Autodesk Inventor part; units mm, degrees
ref_plane "YZ Plane" through (0, 0, 0) normal (1, 0, 0) x (0, 1, 0)
ref_plane "XZ Plane" through (0, 0, 0) normal (0, 1, 0) x (-1, 0, 0)
ref_plane "XY Plane" through (0, 0, 0) normal (0, 0, 1) x (1, 0, 0)
sketch "Skizze1" plane through (0, 0, 0) normal (0, 0, 1) x (1, 0, 0)
  line L0 (11.5, 38) -> (-11.5, 38)
  line L1 (-11.5, 38) -> (-11.5, -38)
  line L2 (-11.5, -38) -> (11.5, -38)
  line L3 (11.5, -38) -> (11.5, 38)
  line L4 (11.5, 38) -> (-11.5, -38) construction
  line L5 (-11.5, 38) -> (11.5, -38) construction
  line L6 (-23, -50) -> (23, -50)
  line L7 (23, -50) -> (23, -38)
  line L8 (23, -38) -> (-23, -38)
  line L9 (-23, -38) -> (-23, -50)
  line L10 (-23, -50) -> (23, -38) construction
  line L11 (23, -50) -> (-23, -38) construction
  line L12 (-23, -38) -> (-11.5, -38)
  line L13 (-11.5, -38) -> (-11.5, 12)
  line L14 (-11.5, 12) -> (-23, 12)
  line L15 (-23, 12) -> (-23, -38)
  line L16 (23, -38) -> (11.5, -38)
  line L17 (11.5, -38) -> (11.5, 12)
  line L18 (11.5, 12) -> (23, 12)
  line L19 (23, 12) -> (23, -38)
  point P0 (0, 0)
  point P1 (0, -44)
  point P2 (0, -38)
  dimension "d0" = 23
  dimension "d1" = 76
  dimension "d2" = 12
  dimension "d3" = 50
  dimension "d4" = 50
  dimension "d5" = 46
extrude "Extrusion1" add sketch "Skizze1" along normal blind 10 contours L18 L19 L8 L3 | L1 L8 L15 L14 | L8 L7 L6 L9 L2
sketch "Skizze2" plane through (-11.5, -38, 0) normal (1, 0, 0) x (0, 0, -1)
  line L0 (0, 50) -> (0, -12)
  line L1 (0, -7.7211) -> (-0.5, -7.7211)
  line L2 (-0.5, -7.7211) -> (-2, -3.621)
  line L3 (-2, -3.621) -> (-2, 50)
  line L4 (-2, 50) -> (0, 50)
  line L5 (0, 0) -> (0, 50)
  point P0 (0, 38)
  point P1 (0, 5.0638)
  dimension "d8" = 0.5
  dimension "d15" = 2
extrude "Extrusion2" cut sketch "Skizze2" along normal blind 25 and the other way blind 2
sketch "Skizze3" plane through (-23, -50, 0) normal (-1, 0, 0) x (0, 0, 1)
  line L0 (0, 62) -> (0, 0)
  line L1 (0, 0) -> (10, 0)
  line L2 (10, 62) -> (10, 0)
  line L3 (0, 62) -> (10, 62)
  circle A0 centre (6.7241, 56.1881) radius 1.5
  point P0 (0, 50)
  dimension "d11" = 3
extrude "Extrusion3" cut sketch "Skizze3" against normal through all contours A0
fillet "Rundung1" radius 2 4 edges at (17.25, 12, 10) (-17.25, 12, 10) (-23, -50, 5) (23, -50, 5)
sketch "Skizze4" plane through (0, 0, 0) normal (0, 0, -1) x (-1, 0, 0)
  arc A0 (-23, -48) -> (-21, -50) centre (-21, -48) ccw
  line L0 (21, -50) -> (-21, -50)
  arc A1 (21, -50) -> (23, -48) centre (21, -48) ccw
  line L1 (23, 12) -> (23, -48)
  line L2 (13.5, 12) -> (23, 12)
  line L3 (13.5, 12) -> (13.5, -45.7211)
  line L4 (13.5, -45.7211) -> (-13.5, -45.7211)
  line L5 (-13.5, -45.7211) -> (-13.5, 12)
  line L6 (-23, 12) -> (-13.5, 12)
  line L7 (-23, -48) -> (-23, 12)
  line L8 (-25, 14) -> (-11.5, 14)
  line L9 (-11.5, 14) -> (-11.5, -43.7211)
  line L10 (-11.5, -43.7211) -> (11.5, -43.7211)
  line L11 (11.5, -43.7211) -> (11.5, 14)
  line L12 (11.5, 14) -> (25, 14)
  line L13 (25, 14) -> (25, -48)
  arc A2 (21, -52) -> (25, -48) centre (21, -48) ccw
  line L14 (21, -52) -> (-21, -52)
  arc A3 (-25, -48) -> (-21, -52) centre (-21, -48) ccw
  line L15 (-25, -48) -> (-25, 14)
  line L16 (-23, 12) -> (-25, 12)
  line L17 (23, 12) -> (25, 12)
  point P0 (0, 0)
  dimension "d18" = 2
extrude "Extrusion4" add sketch "Skizze4" against normal blind 2 contours A0 L0 A1 L1 L17 L13 A2 L14 A3 L15 L16 L7
sketch "Skizze5" plane through (0, 0, 10) normal (0, 0, 1) x (1, 0, 0)
  arc A0 (21, -50) -> (23, -48) centre (21, -48) ccw
  line L0 (23, -48) -> (23, 10)
  line L1 (11.5, 10) -> (23, 10)
  line L2 (11.5, 10) -> (11.5, -38)
  line L3 (11.5, -38) -> (-11.5, -38)
  line L4 (-11.5, -38) -> (-11.5, 10)
  line L5 (-23, 10) -> (-11.5, 10)
  line L6 (-23, 10) -> (-23, -48)
  arc A1 (-23, -48) -> (-21, -50) centre (-21, -48) ccw
  line L7 (-21, -50) -> (21, -50)
  line L8 (-17.3893, -44.3893) -> (-17.3893, 4.3893)
  line L9 (-17.3893, 4.3893) -> (-17.1107, 4.3893)
  line L10 (-17.1107, 4.3893) -> (-17.1107, -43.6107)
  line L11 (-17.1107, -43.6107) -> (17.1107, -43.6107)
  line L12 (17.1107, -43.6107) -> (17.1107, 4.3893)
  line L13 (17.1107, 4.3893) -> (17.3893, 4.3893)
  line L14 (17.3893, 4.3893) -> (17.3893, -44.3893)
  line L15 (17.3893, -44.3893) -> (-17.3893, -44.3893)
  point P0 (0, 0)
hole "Bohrung1" at (-17.3893, -44.3893, 10) at (17.3893, -44.3893, 10) at (17.3893, 4.3893, 10) at (-17.3893, 4.3893, 10) direction (0, 0, -1) diameter 2.8 depth 12 tip angle 118
properties part number "Anglerfish_coverslipclamp_top"
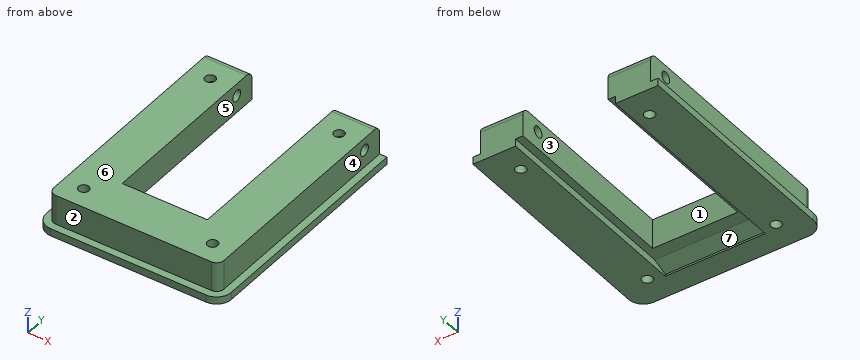
Source: CAD feature listing. Evaluate the final solid. Frame: model axes, mm. Face numbers are marked on the shaded views. A direction names the side the tool comes from. Coordinates: 2 decimals unless noted, no trailing zeros. Loops run counter-clockwise (first coordinate to the right, second up) from the corner with the lowest first, then second, coordinate; pieces in that order, holes last. Notation, with made-up numbers: M 12.5,-10.5 L 29.5,-10.5 A28 ccw 29.5,7.5 Z; hole C 23.5,-27 d11. An arc over 180 degrees is marked long. Use a Markdown table: item, result. Add a question column.
Q1. Section query A-A, the plane z = 6. Return loops of the section in (x, y), and give its area (3 significant figures).
Q2. Section query C-C, the plane x = 0.5. Return loops of the section in (y, z).
Q3. Access query for the marked faces 5, 6 and 7. Directions: +Z, -Z, +X, -X, +Y, -Y. A direction counts if a zero-diameter tool reaches every point of the face in a straight line with its end or side. Return the directions, or none.
Q4. Material intervals for L1, parallel to Y at x = -17.5, z = 3.5; L2, parallel to X at y = -44.5, z = 6.25; L3, parallel to X at y = -10.5, z = 6.25, sorted ascending.
Q5. Draft query along X for the marked faces 1, 2, 3 and 4. Return one class per face: pulls with the +X half, pulls with the -X half, needs draft (parallel to the pull), parting line crosses it, or undercut.
Q6. Section query B-B, the plane y = -22.5. Return loops of the section in (x, z).
Q7. Section query D-D, the plane y = -46.5. Return loops of the section in (x, z).
Q8. First-contact query: pin 1 (2.5 mm diameter, centred on y = -27, z = 7.5, fed in from +X); pin 2 (1.5 mm diameter, centred on x = 6.5, z = 5.5, fed in from +Y); pin 3 (13.5 mm diameter, centred on x = 4, y = -26, fed in from -Z); pin 4 (5 mm diameter, centred on y = 6.19, z = 6.72, fed in from -X). Flat tips, straight axial feed; report the tip coordinate or a pass-through.
Result:
| question | item | result |
|---|---|---|
| 1 | outline | M -23,-48 A2 ccw -21,-50 L 21,-50 A2 ccw 23,-48 L 23,4.87 L 18.7,4.87 A1.4 cw long 16.08,4.87 L 11.5,4.87 L 11.5,-38 L -11.5,-38 L -11.5,4.87 L -16.08,4.87 A1.4 cw long -18.7,4.87 L -23,4.87 Z; M -23,7.5 L -11.5,7.5 L -11.5,12 L -23,12 Z; M 11.5,7.5 L 23,7.5 L 23,12 L 11.5,12 Z; hole C -17.39,-44.39 d2.8; hole C 17.39,-44.39 d2.8 |
| 1 | area | 1,620 mm2 |
| 2 | outline | M -52,0 L -45.72,0 L -45.72,0.5 L -41.62,2 L -38,2 L -38,10 L -50,10 L -50,2 L -52,2 Z |
| 3 | face 5 | +Z, -Z, +Y |
| 3 | face 6 | +Z, +X, -X, +Y, -Y |
| 3 | face 7 | -Z, +Y |
| 4 | L1 | y = -50 to -45.78, -42.99 to 2.99, 5.78 to 12 |
| 4 | L2 | x = -23 to -18.78, -15.99 to 15.99, 18.78 to 23 |
| 4 | L3 | x = -23 to -11.5, 11.5 to 23 |
| 5 | face 1 | undercut |
| 5 | face 2 | needs draft |
| 5 | face 3 | undercut |
| 5 | face 4 | pulls with the +X half |
| 6 | outline | M -25,0 L -13.5,0 L -13.5,2 L -11.5,2 L -11.5,10 L -23,10 L -23,2 L -25,2 Z; M 11.5,2 L 13.5,2 L 13.5,0 L 25,0 L 25,2 L 23,2 L 23,10 L 11.5,10 Z |
| 7 | outline | M -25,0 L 25,0 L 25,2 L 23,2 L 23,10 L -23,10 L -23,2 L -25,2 Z |
| 8 | pin 1 | stops at x = 23 |
| 8 | pin 2 | stops at y = -38 |
| 8 | pin 3 | passes through |
| 8 | pin 4 | stops at x = -23 |
